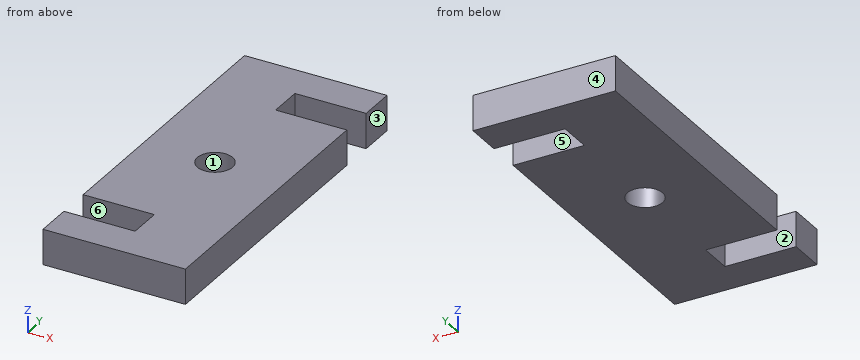
```python
from build123d import *

# Parameters (mm, degrees)
SKETCH012_R = 2.5
PAD_DEPTH   = 5


with BuildPart() as part:
    # Sketch012 → Pad (new body)
    with BuildSketch(Plane(origin=(0, -5, 100), x_dir=(1, 0, 0), z_dir=(0, 0, 1))):
        Polygon((-10.1, 25.1), (10.1, 25.1), (10.1, 19.9), (0, 19.9), (0, 15.1), (10.1, 15.1), (10.1, -25.1), (-10.1, -25.1), (-10.1, -19.9), (0, -19.9), (0, -15.1), (-10.1, -15.1), align=None)
        Circle(SKETCH012_R, mode=Mode.SUBTRACT)
    extrude(amount=PAD_DEPTH)


solid = part.part
```
Part model, mm, in its own coordinate system. Face numbers are marked on the shaded views. A direction names the side the tool comes from. Round coordinates to 2 decimals unless told otherwise and drop trailing zeros. Loops run counter-clockwise (first coordinate to the right, second up) from the corner with the lowest first, then second, coordinate; pieces in that order, holes last. Notation, with made-up numbers: (47, -24.75) -> (99, -24.75) arc R35 ccw to (99, 7.25) -> close; hole circle Ø4 at (27.5, 50). An arc over 180 degrees is marked (long way). Use CSV: the item, a comma, the result in double quotes. Start each with the question number.
1) Pull direction X, two halves, no side cores. Call the marked faces 1, 2 and 3: +X half, -X half, draft (parallel to the pull), parting line (faces both ways), or undercut.
2) Cut at C-C, the plane x = -1.25. Write the cut outline in (y, z).
3) Cut at D-D, the plane y = 14. Write the cut outline in (x, z).
4) Cut at B-B, the plane z = 101.15. Write the cut outline in (x, y).
5) Drop flat-ended pins along their axis: P1, Ø2.5, axis at y = -22, z = 102.5, coming from the -X side; P2, Ø3, axis at x = 0, y = -5, coming from the +Z side; P3, Ø1.5, axis at y = 12, z = 102.5, coming from the +X side. Give the stop position or say it passes through.
6) Wall check: L1, parallel to Y at x = -4, z = 100.75; L2, parallel to Y at x = 9, z = 102.65; L3, parallel to Y at x = 2, z = 102.55. Give the ranges that are in metal, low to high. Write a range as [from, to].
7) Cut at A-A, the plane y = -5. Write the cut outline in (x, z).
8) Which spindle directions (+Z, -Z, +X, -X, +Y, -Y) get a long thin tool onto all of the face, cutting with end or side? Do the marked faces 4, 5 and 6. Say none if no direction does.
Determined:
1,face 1,"undercut"
1,face 2,"draft"
1,face 3,"+X half"
2,outline,"(-30.1, 100) -> (-24.9, 100) -> (-24.9, 105) -> (-30.1, 105) -> close; (-20.1, 100) -> (-7.17, 100) -> (-7.17, 105) -> (-20.1, 105) -> close; (-2.83, 100) -> (20.1, 100) -> (20.1, 105) -> (-2.83, 105) -> close"
3,outline,"(-10.1, 100) -> (0, 100) -> (0, 105) -> (-10.1, 105) -> close"
4,outline,"(-10.1, -30.1) -> (10.1, -30.1) -> (10.1, 10.1) -> (0, 10.1) -> (0, 14.9) -> (10.1, 14.9) -> (10.1, 20.1) -> (-10.1, 20.1) -> (-10.1, -20.1) -> (0, -20.1) -> (0, -24.9) -> (-10.1, -24.9) -> close; hole circle Ø5 at (0, -5)"
5,P1,"stops at x = 0"
5,P2,"passes through"
5,P3,"stops at x = 0"
6,L1,"y = [-30.1, -24.9], [-20.1, 20.1]"
6,L2,"y = [-30.1, 10.1], [14.9, 20.1]"
6,L3,"y = [-30.1, -6.5], [-3.5, 10.1], [14.9, 20.1]"
7,outline,"(-10.1, 100) -> (-2.5, 100) -> (-2.5, 105) -> (-10.1, 105) -> close; (2.5, 100) -> (10.1, 100) -> (10.1, 105) -> (2.5, 105) -> close"
8,face 4,"+Z, -Z, +X, -X, +Y"
8,face 5,"+Z, -Z, +X"
8,face 6,"+Z, -Z, -X"
